Model file for the job. Use its own axes, mm. Face numbers are marked on the shaded views. A direction names the side the tool comes from. Coordinates: 2 decimals unless noted, no trailing zeros. Loops run counter-clockwise (first coordinate to the right, second up) from the corner with the lowest first, then second, coordinate; pieces in that order, holes last. Notation, with made-up numbers: (52, 83.5) - (84, 83.5) arc R28 ccw to (84, 109.5) - close; hole circle Ø7 at (-25.75, 49.25). An arc over 180 degrees is marked (long way). Write each question's results on one line, items separated by ' | '. Start each with the question number.
```python
from build123d import *

# Parameters (mm, degrees)
CROQUIS1_W              = 6
CROQUIS1_H              = 6
SALIENTE_EXTRUIR1_DEPTH = 3.5
CROQUIS2_R              = 4.5
SALIENTE_EXTRUIR2_DEPTH = 4
CROQUIS3_R              = 3.75
SALIENTE_EXTRUIR3_DEPTH = 5


with BuildPart() as part:
    # Croquis1 → Saliente-Extruir1 (new body)
    with BuildSketch(Plane.XY):
        Rectangle(CROQUIS1_W, CROQUIS1_H)
    extrude(amount=SALIENTE_EXTRUIR1_DEPTH)

    # Croquis2 → Saliente-Extruir2 (add)
    with BuildSketch(Plane.XY.offset(3.5)):
        Circle(CROQUIS2_R)
    extrude(amount=SALIENTE_EXTRUIR2_DEPTH)

    # Croquis3 → Saliente-Extruir3 (add)
    with BuildSketch(Plane.XY.offset(7.5)):
        Circle(CROQUIS3_R)
    extrude(amount=SALIENTE_EXTRUIR3_DEPTH)


solid = part.part
```
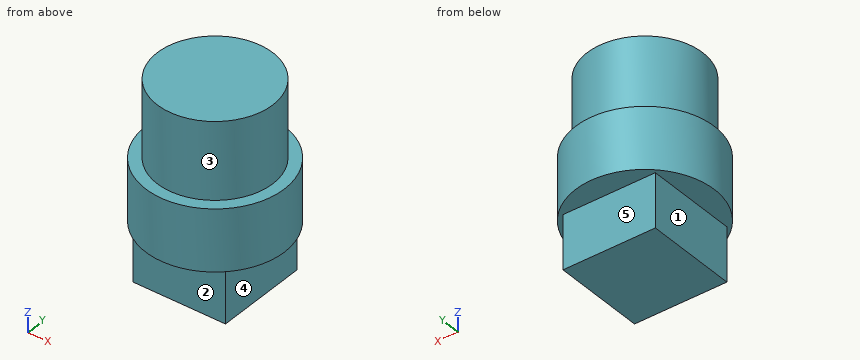
Q1. Cut at B-B (x = -3.5). List the corners of the cut face in (y, z).
Q2. Cut at C-C (z = 7.75). List the corners of the cut face in (x, y), and give its area (3 significant figures).
Q3. Pin check, flat tips, straight feed: pin 1 (1 mm diameter, centred on x = 0, z = 1.5, fed in from -Y); pin 2 (3 mm diameter, centred on x = 3.5, z = 8.5, fed in from -Y); pin 3 (1.5 mm diameter, centred on x = -3, z = 6.5, fed in from +Y). Stop position of each tip, or through.
Q4. Which spindle directions (+Z, -Z, +X, -X, +Y, -Y) get a long thin tool onto all of the face, cutting with end or side? Do the marked faces 1, 2, 3, 4 and 5. Say none if no direction does.
Q5. Cut at A-A (y = 0). List the corners of the cut face in (x, z), and give its area (3 significant figures).
Q6. Drill centre lines: L1, parallel to X at y = 2.25, z = 8; L2, parallel to Z at x = -3.75, y = 1. Where is each one in solid material? Low to high. Write a range as from..to.
Check result:
1) outline: (-2.83, 3.5) - (2.83, 3.5) - (2.83, 7.5) - (1.35, 7.5) - (1.35, 12.5) - (-1.35, 12.5) - (-1.35, 7.5) - (-2.83, 7.5) - close
2) outline: circle Ø7.5 at (0, 0) | area: 44.2 mm²
3) pin 1: y = -3 | pin 2: y = -3.82 | pin 3: y = 3.9
4) face 1: -Z, -X, +Y, -Y | face 2: -Z, +X, -X, -Y | face 3: +Z | face 4: -Z, +X, +Y, -Y | face 5: -Z, +X, -X, +Y
5) outline: (-4.5, 3.5) - (-3, 3.5) - (-3, 0) - (3, 0) - (3, 3.5) - (4.5, 3.5) - (4.5, 7.5) - (3.75, 7.5) - (3.75, 12.5) - (-3.75, 12.5) - (-3.75, 7.5) - (-4.5, 7.5) - close | area: 94.5 mm²
6) L1: -3..3 | L2: 3.5..7.5
